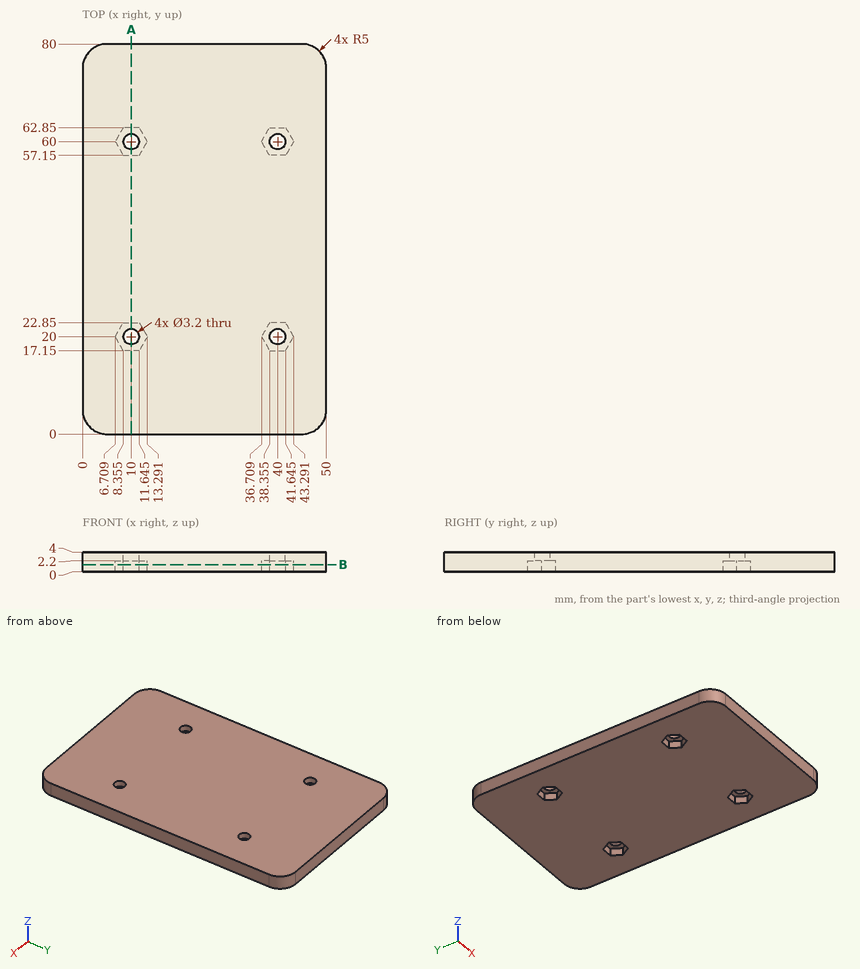
Input: dimensioned drawing with shaded views. Units: mm. Origin: part minimum x, y, z. Coordinates: 2 decimals unless noted, no trailing zeros. Order: outer loops, then holes, each group sorted by start corner. A loop starts at its lowest first (then second) coordinate and runs counter-clockwise, first axis right, second up.
1. Cut plane B-B, the plane z = 1.45. Count the separate pieces of the cut face and the enclosed holes in it, plus the area to 3 significant figures.
Checked values:
separate pieces: 1
enclosed holes: 4
area: 3,870 mm2
2. Contact query for a flat-ended pin moving along its axis: P1, Ø4, axis at x = 10, y = 20, coming from the -Z side. Output: stop coordinate, or through.
Checked values:
P1: stops at z = 2.2
3. Cut plane A-A, the plane x = 10. Return loops of the section in (y, z).
Checked values:
outline: (0, 0) - (17.15, 0) - (17.15, 2.2) - (18.4, 2.2) - (18.4, 4) - (0, 4) - close; (21.6, 2.2) - (22.85, 2.2) - (22.85, 0) - (57.15, 0) - (57.15, 2.2) - (58.4, 2.2) - (58.4, 4) - (21.6, 4) - close; (61.6, 2.2) - (62.85, 2.2) - (62.85, 0) - (80, 0) - (80, 4) - (61.6, 4) - close
4. Ray query, line 1 along Y through (x, z) = (10.5, 0.55); line 2 along Y through (x, z) = (40, 2.75); line 3 along X through (y, z) = (60.5, 3.75). Return the intervals inside material, ascending.
Checked values:
line 1: y = 0 to 17.15, 22.85 to 57.15, 62.85 to 80
line 2: y = 0 to 18.4, 21.6 to 58.4, 61.6 to 80
line 3: x = 0 to 8.48, 11.52 to 38.48, 41.52 to 50
